For this review, use the dimensioned drawing (mm, ordinates from the lowest corner) and the shaded views. Coordinates: 2 decimals unless noted, no trailing zeros. Write each loop counter-clockwise with the first axis right and the second up, starting at its lowest first coordinate (ties: lowest second). Pieces come first, ordered by that corner, then holes.
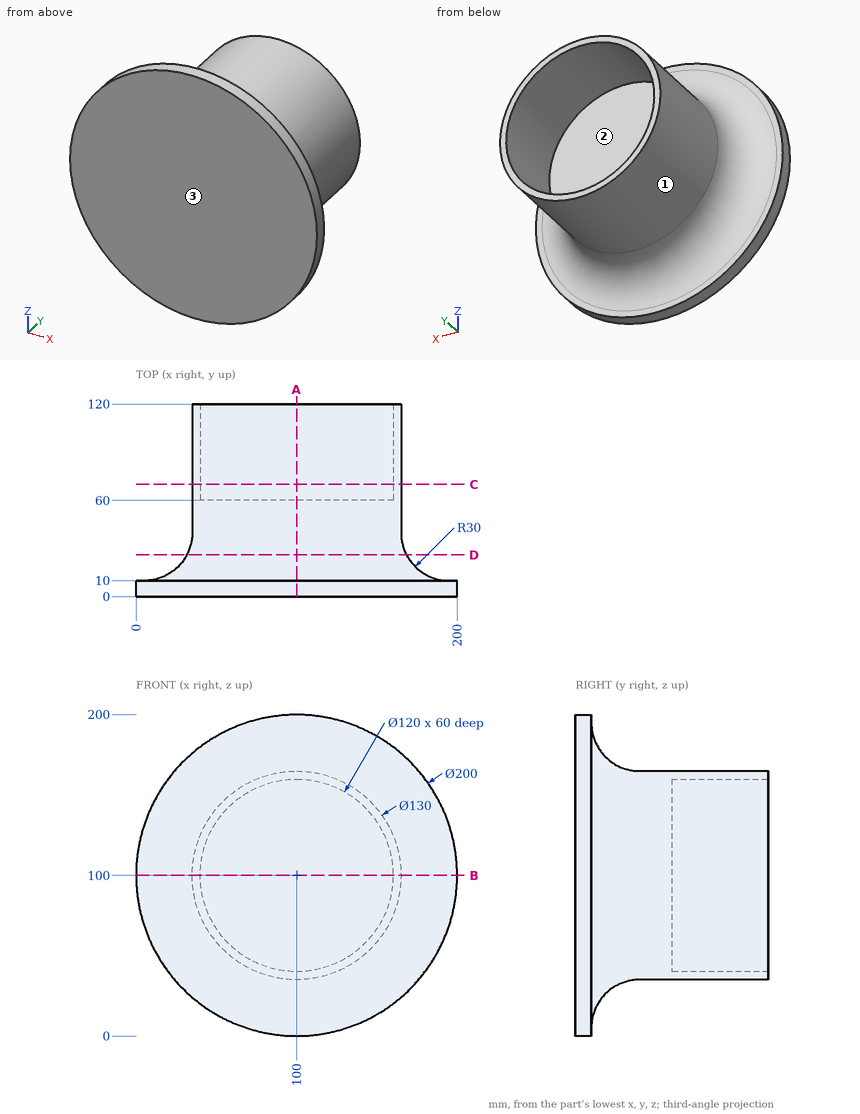
(1) Consider section C-C (y = 70). Give the boundary of the cut face in (x, z), plus the area to 3 significant figures.
(2) Consider section D-D (y = 26). Give the boundary of the cut face in (x, z).
(3) Consider section A-A (x = 100). Give the boundary of the cut face in (y, z).
(4) Consider section B-B (z = 100). Give the boundary of the cut face in (x, y), plus the area to 3 significant figures.
(5) Mouldability with a two-part tool opening along Z and no side actions: class the marked faces 1, 2 and 3 as +Z half, -Z half, draft (parallel to the pull), parting line (faces both ways), or undercut.
(6) Insertion check: pin 1 Ø6 at (x, y) = (83.5, 76.5) entering from +Z; pin 2 Ø12 at (x, z) = (152.5, 89) entering from +Y; pin 3 Ø6 at (x, y) = (85.5, 65.5) entering from -Z. Each pin has a flat end and moves straight along its axis. Give the tip position at first contact, or say it passes through.
(7) Wall thickness on line 1 (X direction, y = 96, z = 100); line 2 (X direction, y = 115, z = 102.5); line 3 (Y direction, x = 121, z = 110.5): over which ranges is each line inside the solid? List them lowest first.
Results:
1. outline: circle Ø130 at (100, 100); hole circle Ø120 at (100, 100)
1. area: 1,960 mm2
2. outline: circle Ø136.93 at (100, 100)
3. outline: (0, 0) - (10, 0) - (10, 5) arc R30 cw to (40, 35) - (120, 35) - (120, 40) - (60, 40) - (60, 160) - (120, 160) - (120, 165) - (40, 165) arc R30 cw to (10, 195) - (10, 200) - (0, 200) - close
4. outline: (0, 0) - (200, 0) - (200, 10) - (195, 10) arc R30 cw to (165, 40) - (165, 120) - (160, 120) - (160, 60) - (40, 60) - (40, 120) - (35, 120) - (35, 40) arc R30 cw to (5, 10) - (0, 10) - close
4. area: 9,490 mm2
5. face 1: parting line
5. face 2: undercut
5. face 3: draft
6. pin 1: stops at z = 163.58
6. pin 2: stops at y = 60
6. pin 3: stops at z = 36.03
7. line 1: x = 35 to 40, 160 to 165
7. line 2: x = 35.05 to 40.05, 159.95 to 164.95
7. line 3: y = 0 to 60
